Geometry: see drawing. Coordinates: mm, zero at the bounding-box minimum. Coordinates: 2 decimals unless noted, no trailing zeros. Loops run counter-clockwise (first coordinate to the right, second up) from the corner with the lowest first, then second, coordinate; pieces in that order, holes last.
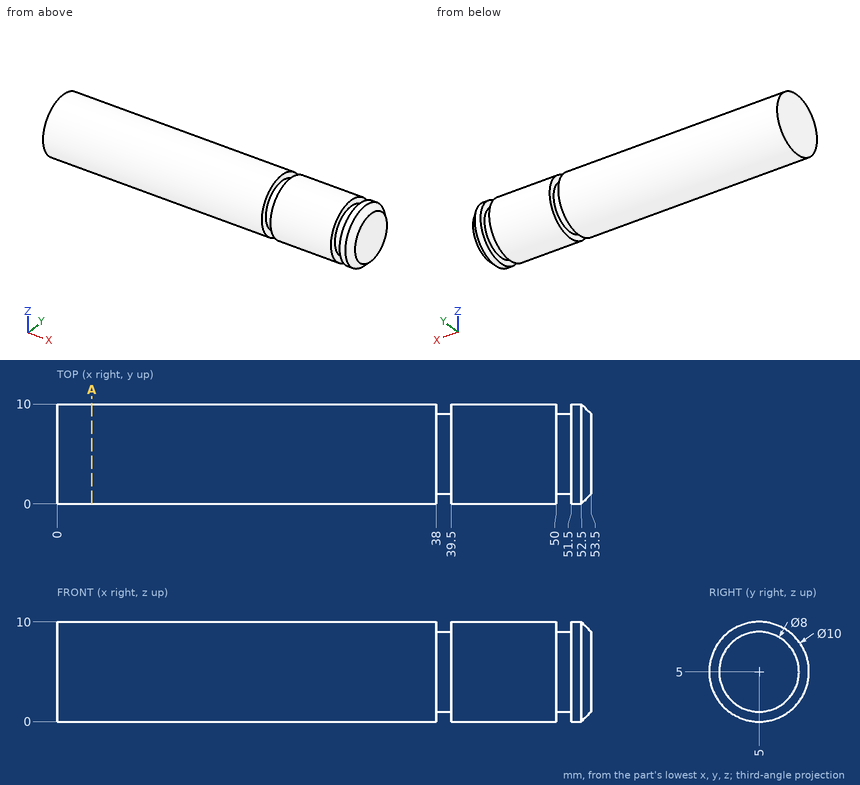
Item 1: Line query: L1, parallel to X at y = 4, z = 9.5; L2, parallel to Y at x = 10, z = 2. Output: solid intervals per line, ascending.
Result:
L1: x = 0 to 38, 39.5 to 50, 51.5 to 52.89
L2: y = 1 to 9
Item 2: Section query A-A (x = 3.5). Output: boundary loops of the cut face in (y, z).
Result:
outline: circle Ø10 at (5, 5)
Item 3: Contact query for flat-ended pins moving along their axis: P1, Ø4, axis at x = 16, y = 7.5, coming from the -Z side; P2, Ø4, axis at x = 38, z = 4, coming from the -Y side; P3, Ø3, axis at x = 44, y = 7, coming from the +Z side. Output: stop coordinate, or through.
Result:
P1: stops at z = 0.03
P2: stops at y = 0
P3: stops at z = 9.97
